CAD build for the part. Positions are in the model's coordinates, mm. Face numbers are marked on the shaded views. A direction names the side the tool comes from. Give positions to 0.01 mm unless a question says otherwise; leave off trailing zeros. Write each loop counter-clockwise with the first axis right and the second up, starting at its lowest first coordinate (ties: lowest second). Pieces come first, ordered by that corner, then holes. Notation, with made-up numbers: (22.5, 57.5) -> (74.5, 57.5) arc R7 cw to (74.5, 64.5) -> close; hole circle Ø1 at (10, -5.5). An arc over 180 degrees is marked (long way). Answer in a Markdown table with one row per item. Add a question column.
```python
from build123d import *

# Parameters (mm, degrees)
SKETCH3_W                  = 9.525
SKETCH3_H                  = 10.795
SKETCH10_R                 = 1.1811
CUT_EXTRUDE1_DEPTH         = 17.51
CHAMFER1_SIZE              = 0.381
F_10_24_TAPPED_HOLE1_D     = 3.7973
F_10_24_TAPPED_HOLE1_DEPTH = 6.35
F_10_24_TAPPED_HOLE1_TIP   = 1.140824014


with BuildPart() as part:
    # Sketch3 → Revolve1 (revolve)
    with BuildSketch(Plane.XY, mode=Mode.PRIVATE) as revolve1_sk:
        with Locations((-4.7625, 11.1125)):
            Rectangle(SKETCH3_W, SKETCH3_H)
    revolve(revolve1_sk.sketch.rotate(Axis((0, 5.715, 0), (0, 1, 0)), 180), axis=Axis((0, 5.715, 0), (0, 1, 0)))  # turned: the seam where the file's is

    # Sketch10 → Cut-Extrude1 (cut, through all)
    with BuildSketch(Plane(origin=(0, 0, 0), x_dir=(1, 0, 0), z_dir=(0, 1, 0))):
        with Locations(Location((0, -7.239, 0), (0, 0, 180))):  # turned: the seam where the file's is
            Circle(SKETCH10_R)
    extrude(amount=CUT_EXTRUDE1_DEPTH, mode=Mode.SUBTRACT)

    # Chamfer1
    chamfer1_edges = [part.edges().sort_by_distance(p)[0] for p in [
        (-9.525, 16.51, 0),
        (-9.525, 5.715, 0),
    ]]
    chamfer(chamfer1_edges, length=CHAMFER1_SIZE)

    # #10-24 Tapped Hole1
    with Locations(Plane(origin=(0, 16.51, 0), x_dir=(1, 0, 0), z_dir=(0, 1, 0))):
        with Locations((0, 0)):
            Hole(F_10_24_TAPPED_HOLE1_D / 2, depth=F_10_24_TAPPED_HOLE1_DEPTH)
            with Locations((0, 0, -(F_10_24_TAPPED_HOLE1_DEPTH + F_10_24_TAPPED_HOLE1_TIP / 2))):  # 118° drill point
                Cone(0, F_10_24_TAPPED_HOLE1_D / 2, F_10_24_TAPPED_HOLE1_TIP, mode=Mode.SUBTRACT)

    # Sketch15 → Cut-Revolve3 (revolve, cut)
    with BuildSketch(Plane.XY):
        with BuildLine():
            Line((-11.578836277, 15.257357798), (-11.578836277, 2.536311926))
            Line((-11.578836277, 2.536311926), (1.226518223, 2.536311926))
            ThreePointArc((1.226518223, 2.536311926), (-5.290998219, 8.781234574), (-11.578836277, 15.257357798))
        make_face()
    cut_revolve3 = revolve(axis=Axis((170.909475954, 186.149475954, 0), (0, -1, 0)), mode=Mode.SUBTRACT)

    # Mirror2: Cut-Revolve3 across plane
    add(cut_revolve3.mirror(Plane(origin=(0, 0, 0), x_dir=(0, 0, 1), z_dir=(1, 0, 0))), mode=Mode.SUBTRACT)

    # Sketch16 → Cut-Revolve4 (revolve, cut)
    with BuildSketch(Plane.XY):
        Polygon((0, 16.999184369), (0, 16.129), (5.08, 16.129), (6.340889503, 17.389889503), align=None)
    revolve(axis=Axis((0, 0, 0), (0, 1, 0)), mode=Mode.SUBTRACT)


solid = part.part
```
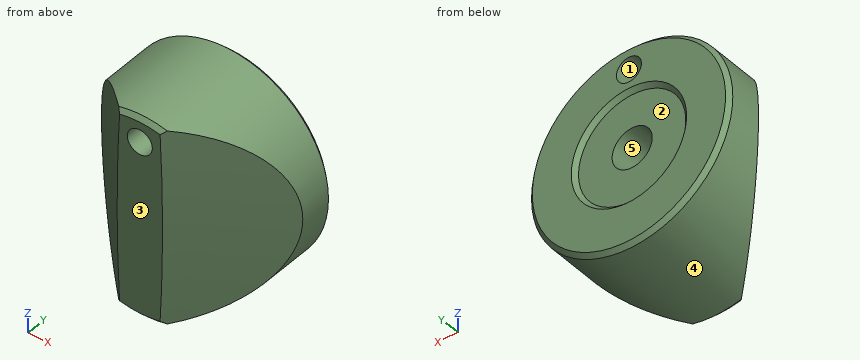
Item 1: Probe L1, parallel to Z at x = 0, y = 12.8 (3 decimals); L2, parallel to Z at x = 0.25, y = 9.75; L3, parallel to Y at x = 0.75, z = -2.5 (3 decimals). List the from-to ranges inside material, lowest first. Write a range as from..to.
Item 2: Slice it at A-A, the plane y = 11. State how many separate pieces and enclosed holes the cut face has, then the cut area to 3 significant figures.
Item 3: Drop flat-ended pins along their axis: pin 1 Ø2 at (y, z) = (15, 3) entering from -X; pin 2 Ø3 at (x, z) = (-1.5, 1) entering from +Y; pin 3 Ø3 at (x, y) = (-7.5, 14.5) entering from +Z. Give the stop position or say it passes through.
Item 4: Which spindle directions (+Z, -Z, +X, -X, +Y, -Y) get a long thin tool onto all of the face, cutting with end or side? Do the marked faces 1 and 2. Say none if no direction does.
Item 5: Mould opens along Z. For the marked faces 3, 4 and 5 say: released by +Z, released by -Z, zero draft, split by the parting line, or undercut.
Item 6: Slice it at B-B, the plane y = 14. List the corners of the cut face in (x, z) (3 decimals).
Answer key:
| question | item | result |
|---|---|---|
| 1 | L1 | z = -9.525..-1.899, 1.899..6.058, 8.42..9.525 |
| 1 | L2 | z = -9.52..-1.19, 1.19..6.08, 8.39..9.52 |
| 1 | L3 | y = 5.715..16.129 |
| 2 | separate pieces | 1 |
| 2 | enclosed holes | 2 |
| 2 | area | 236 mm² |
| 3 | pin 1 | stops at x = -9.31 |
| 3 | pin 2 | stops at y = 16.13 |
| 3 | pin 3 | stops at z = 7.4 |
| 4 | face 1 | +Y, -Y |
| 4 | face 2 | +Y |
| 5 | face 3 | zero draft |
| 5 | face 4 | split by the parting line |
| 5 | face 5 | undercut |
| 6 | outline | circle Ø19.05 at (0, 0); hole circle Ø3.797 at (0, 0); hole circle Ø2.362 at (0, 7.239) |
